Geometry check sheet. Reference: the model listing, model coordinates, mm. Face numbers are marked on the shaded views. A direction names the side the tool comes from. Round coordinates to 2 decimals unless told otherwise and drop trailing zeros. Order: outer loops, then holes, each group sorted by start corner. A loop starts at its lowest first (then second) coordinate and runs counter-clockwise, first axis right, second up. Notation, with made-up numbers: M -3,-35 L 8,-35 A13 ccw 8,-12 Z; hole C -13,-12 d3. An arc over 180 degrees is marked long. Answer as a JSON object with one key per item and string values. Group by question number.
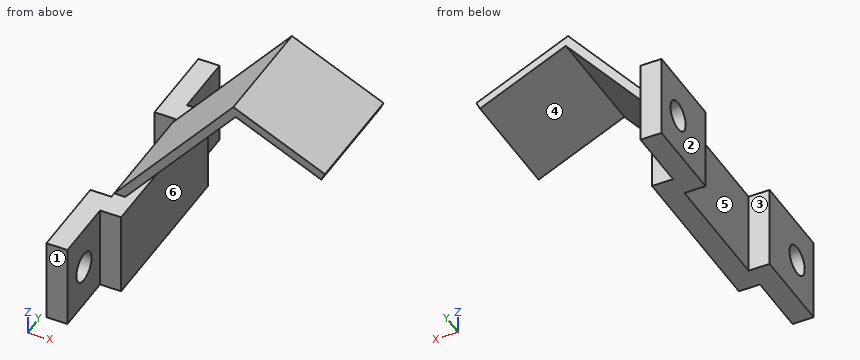
```python
from build123d import *

# Parameters (mm, degrees)
F1_DEPTH = 10
F2_DEPTH = 6.75
F0_W     = 2.5
F0_H     = 10
F3_DEPTH = 17.5
F4_DEPTH = 7.375
F5_R     = 1.75
F6_DEPTH = 5


with BuildPart() as f1:
    # F0 (on Front) → F1 (new body, symmetric)
    with BuildSketch(Plane.XZ):
        Polygon((1.25, -5), (1.25, 5), (0.055407, 5), (-1.25, 5), (-1.25, -5), align=None)
    extrude(amount=F1_DEPTH, both=True)

    # F0 (on Front) → F2 (join, symmetric)
    with BuildSketch(Plane.XZ):
        Polygon((-1.25, 5), (0.055407, 5), (13.164144, 20.622384), (23.344403, 15.875251), (23.767021, 16.781559), (12.891327, 21.852978), align=None)
    extrude(amount=F2_DEPTH, both=True)

    # F0 (on Front) → F3 (join, symmetric)
    with BuildSketch(Plane.XZ):
        with Locations((-2.5, 0)):
            Rectangle(F0_W, F0_H)
    extrude(amount=F3_DEPTH, both=True)

    # F0 (on Front) → F4 (cut, symmetric)
    with BuildSketch(Plane.XZ):
        with Locations((-2.5, 0)):
            Rectangle(F0_W, F0_H)
    extrude(amount=F4_DEPTH, both=True, mode=Mode.SUBTRACT)

    # F5 (on Right) → F6 (cut, symmetric)
    with BuildSketch(Plane.YZ):
        with Locations((-13.7, 0)):
            Circle(F5_R)
        with Locations((13.7, 0)):
            Circle(F5_R)
    extrude(amount=F6_DEPTH, both=True, mode=Mode.SUBTRACT)


solid = f1.part
```
1) Thickness scan on line 1 along Z through (x, y) = (-1.8, -13.7); line 2 along X through (y, z) = (-3.5, 3.5); line 3 along X through (y, z) = (-15, 2.25). Record the ranges inside material, lowest first. Write a range as [from, to].
2) Go/stop test with flat-tipped pins: P1, Ø1.2, axis at x = -0.5, z = 2, coming from the -Y side; P2, Ø2.5, axis at x = -1.5, y = 6.5, coming from the +Z side; P3, Ø6, axis at y = -12.5, z = 2.5, coming from the +X side. Record where each tip stops, or that it passes through.
3) Sectioned sample at D-D (y = 5). Record the boundary of the cut face in (x, z).
4) Sectioned sample at A-A (z = 0). Record the boundary of the cut face in (x, y) (3 decimals), then the cut area to 3 significant figures.
5) Release check for a two-part mould opening along Y. For the marked faces 1, 2 and 3 record: +Y half, -Y half, draft (parallel to the pull), parting line (faces both ways), or undercut.
6) Sectioned sample at B-B (y = 13.7). Record the boundary of the cut face in (x, z), then the cut area to 4 significant figures.
7) Sectioned sample at C-C (z = 2.75). Record the boundary of the cut face in (x, y) (3 decimals).
8) Set-up check for the marked faces 4, 5 and 6: record each of +Z, -Z, +X, -X, +Y, -Y from which the full face is reachable in a straight line by a thin tool's end or side.
Final values:
{
 "1": {"line 1": "z = [-5, -1.75], [1.75, 5]", "line 2": "x = [-1.25, 1.25]", "line 3": "x = [-3.75, -1.25]"},
 "2": {"P1": "stops at y = -10", "P2": "stops at z = 6.19", "P3": "stops at x = 1.25"},
 "3": {"outline": "M -1.25,-5 L 1.25,-5 L 1.25,5 L 0.06,5 L 13.16,20.62 L 23.34,15.88 L 23.77,16.78 L 12.89,21.85 L -1.25,5 Z"},
 "4": {"outline": "M -3.75,-17.5 L -1.25,-17.5 L -1.25,-15.45 L -3.75,-15.45 Z; M -3.75,-11.95 L -1.25,-11.95 L -1.25,-10 L 1.25,-10 L 1.25,10 L -1.25,10 L -1.25,11.95 L -3.75,11.95 L -3.75,7.375 L -1.25,7.375 L -1.25,-7.375 L -3.75,-7.375 Z; M -3.75,15.45 L -1.25,15.45 L -1.25,17.5 L -3.75,17.5 Z", "area": "83.1 mm^2"},
 "5": {"face 1": "-Y half", "face 2": "draft", "face 3": "undercut"},
 "6": {"outline": "M -3.75,-5 L -1.25,-5 L -1.25,-1.75 L -3.75,-1.75 Z; M -3.75,1.75 L -1.25,1.75 L -1.25,5 L -3.75,5 Z", "area": "16.25 mm^2"},
 "7": {"outline": "M -3.75,-17.5 L -1.25,-17.5 L -1.25,-10 L 1.25,-10 L 1.25,10 L -1.25,10 L -1.25,17.5 L -3.75,17.5 L -3.75,7.375 L -1.25,7.375 L -1.25,-7.375 L -3.75,-7.375 Z"},
 "8": {"face 4": "-Z, +Y, -Y", "face 5": "+Z, -Z, -X", "face 6": "-Z, +X, +Y, -Y"}
}
